Can you work these out from the model? Positions are in its coordinate system, mm. Face numbers are marked on the shaded views. A direction names the side the tool comes from. Coordinates: 2 decimals unless noted, no trailing zeros. Write each loop counter-clockwise with the first axis right and the second up, starting at its lowest first coordinate (ties: lowest second). Pieces come first, ordered by that corner, then holes. Notation, with made-up numbers: (52, 43.5) - (91, 43.5) arc R22 ccw to (91, 71.5) - close; hole circle Ø3 at (57, 66.5). An arc over 180 degrees is marked (long way). Use one line per item in the form item = value. Start each with the question number.
(1) If we section it at B-B on z = -4.5: Please give me the cut outline in (x, y), then the cut area to 3 significant figures.
(2) If we section it at D-D on y = -4.5: Please give me the cut outline in (x, z), then the cut area to 3 significant figures.
(3) Thinking about a two-plate mould opening in Y: for the marked faces 1, 2 and 3, which applies, pulls with the +Y half, pulls with the -Y half, needs draft (parallel to the pull), parting line crosses it, or undercut?
(4) For pin 1 Ø1.6 at (x, z) = (-1.5, -4) entering from -Y; pin 2 Ø3 at (x, y) = (-1, 3) entering from +Z; pin 3 Ø1 at (y, z) = (3, -6) entering from -X, each with a flat end and sliding along its axis, tell me the tip position at first contact or that it passes through.
(5) On a 3-axis mill with a long thin cutter (end or side, diameter ignored), from which of +Z, -Z, +X, -X, +Y, -Y can I reach the whole of each face in a straight line? I mean the marked faces 4, 5 and 6. Say none if no direction works.
(6) If we section it at C-C on y = -23: Please give me the cut outline in (x, z).
(7) If I drill on probe 1 along Y at (x, z) = (2.25, -8.5); probe 2 along Y at (x, z) = (-0.5, -8.75); probe 3 along Y at (x, z) = (6.5, -2.25), over which ranges is the centre line in solid material (lowest first)? Write a range as from..to.
(8) If we section it at A-A on x = 0: Please give me the cut outline in (y, z), then the cut area to 3 significant figures.
```python
from build123d import *

# Parameters (mm, degrees)
SALIENTE_EXTRUIR1_DEPTH = 3
CROQUIS2_W              = 9
CROQUIS2_H              = 4
SALIENTE_EXTRUIR2_DEPTH = 1
CROQUIS3_R              = 7.5
SALIENTE_EXTRUIR3_DEPTH = 2
SALIENTE_EXTRUIR4_START = -3
CROQUIS7_W              = 0.714919667
CROQUIS7_H              = 4
SALIENTE_EXTRUIR4_DEPTH = 6
CROQUIS8_R              = 7.5
SALIENTE_EXTRUIR5_DEPTH = 0.5


with BuildPart() as part:
    # Croquis1 → Saliente-Extruir1 (new body, symmetric)
    with BuildSketch(Plane(origin=(0, 0, 0), x_dir=(0, 0, -1), z_dir=(1, 0, 0))):
        Polygon((0, 0), (0, 4), (9, 4), (8, 3), (1, 3), (1, 0), align=None)
    extrude(amount=SALIENTE_EXTRUIR1_DEPTH, both=True)

    # Croquis2 → Saliente-Extruir2 (add, symmetric)
    with BuildSketch(Plane(origin=(0, 0, 0), x_dir=(0, 0, -1), z_dir=(1, 0, 0))):
        with Locations((4.5, 2)):
            Rectangle(CROQUIS2_W, CROQUIS2_H)
    extrude(amount=SALIENTE_EXTRUIR2_DEPTH, both=True)

    # Croquis3 → Saliente-Extruir3 (add)
    with BuildSketch(Plane.XZ):
        with Locations((0, -4.5)):
            Circle(CROQUIS3_R)
    extrude(amount=SALIENTE_EXTRUIR3_DEPTH)

    # Croquis4 → Revolución1 (revolve)
    with BuildSketch(Plane(origin=(0, 0, 0), x_dir=(0, 0, -1), z_dir=(1, 0, 0))):
        Polygon((-3, -2), (1.475412378, -13), (4.5, -13), (4.5, -2), align=None)
    revolve(axis=Axis((0, -13, -4.5), (0, 1, 0)))

    # Croquis5 → Revolución2 (revolve)
    with BuildSketch(Plane(origin=(0, 0, 0), x_dir=(0, 0, -1), z_dir=(1, 0, 0))):
        with BuildLine():
            Line((4.5, -11), (4.5, -26))
            ThreePointArc((4.5, -26), (-3, -18.5), (4.5, -11))
        make_face()
    revolve(axis=Axis((0, -11, -4.5), (0, -1, 0)))

    # Croquis7 → Saliente-Extruir4 (add)
    with BuildSketch(Plane(origin=(0, 0, 0), x_dir=(0, 0, -1), z_dir=(1, 0, 0)).offset(SALIENTE_EXTRUIR4_START)):
        Polygon((1, 3), (1, 0), (1.204454973, 0), (1.204454973, 2.8), (7.653057768, 2.8), (8, 3), align=None)
        with Locations((-0.357459834, 2)):
            Rectangle(CROQUIS7_W, CROQUIS7_H)
    extrude(amount=SALIENTE_EXTRUIR4_DEPTH)

    # Croquis8 → Saliente-Extruir5 (add)
    with BuildSketch(Plane(origin=(0, 0, 0), x_dir=(1, 0, 0), z_dir=(0, 1, 0))):
        with Locations((0, 4.5)):
            Circle(CROQUIS8_R)
    extrude(amount=SALIENTE_EXTRUIR5_DEPTH)


solid = part.part
```
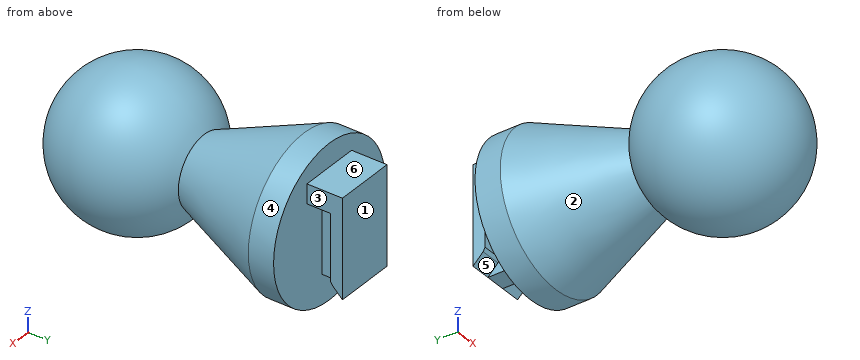
Reported:
q1.outline = (-7.5, -2) - (-3.49, -11.86) arc R7.5 ccw (long way) to (3.49, -11.86) - (7.5, -2) - (7.5, 0.5) - (1, 0.5) - (1, 2.8) - (3, 2.8) - (3, 4) - (-3, 4) - (-3, 2.8) - (-1, 2.8) - (-1, 0.5) - (-7.5, 0.5) - close
q1.area = 330 mm2
q2.outline = circle Ø12.97 at (0, -4.5)
q2.area = 132 mm2
q3.face_1 = pulls with the +Y half
q3.face_2 = undercut
q3.face_3 = needs draft
q4.pin_1 = -25.96
q4.pin_2 = 0.71
q4.pin_3 = -3
q5.face_4 = +Y, -Y
q5.face_5 = -Z, -X
q5.face_6 = +Z, +X, -X, +Y
q6.outline = circle Ø12 at (0, -4.5)
q7.probe_1 = -24.43..-12.57, -9.15..0.5, 3.5..4
q7.probe_2 = -24.66..-12.34, -9.92..4
q7.probe_3 = -21.49..-15.51, -3.53..0.5
q8.outline = (-11.86, -7.99) - (-2, -12) - (0.5, -12) - (0.5, -9) - (4, -9) - (4, 0.71) - (0.5, 0.71) - (0.5, 3) - (-2, 3) - (-11.86, -1.01) arc R7.5 ccw (long way) to start
q8.area = 353 mm2
